Print and shaded views of the part. All mm, measured from the part's lowest x, y and z. A direction names the side the tool comes from. Give positions to 0.01 mm unless a question says otherwise; leave off trailing zeros. Loops run counter-clockwise (first coordinate to the right, second up) from the corner with the lowest first, then second, coordinate; pieces in that order, holes last. Notation, with made-up numbers: M 63.5,62.5 L 90.5,62.5 A22 cw 90.5,99.5 Z; hole C -31,5 d2. An arc over 180 degrees is marked long. Put each result on its own line as item: value. Start each with the question number.
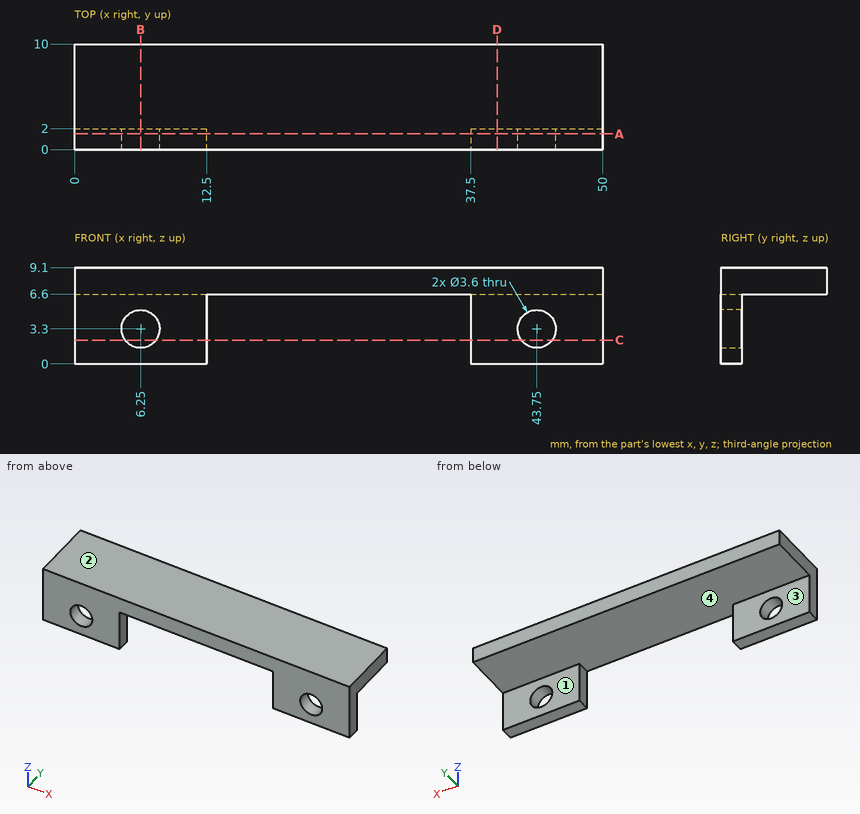
1) Band-saw the part on A-A on y = 1.5. Give the cut face in (x, z).
2) Band-saw the part on D-D on x = 40. Give the cut face in (y, z).
3) Band-saw the part on B-B on x = 6.25. Give the cut face in (y, z).
4) Band-saw the part on C-C on z = 2.25. Give the cut face in (x, y).
5) Wall check: L1, parallel to X at y = 1, z = 6; L2, parallel to Z at x = 6.5, y = 6.75; L3, parallel to Y at x = 4.5, z = 5.75. Give the ranges that are in metal, low to high.
6) Pin check, flat tips, straight feed: pin 1 Ø3 at (x, y) = (19.5, 5) entering from -Z; pin 2 Ø2 at (x, z) = (45, 2.5) entering from +Y. Stop position of each tip, or through.
7) Mould opens along X. For the marked faces 3 and 4 say: +X half, -X half, draft (parallel to the pull), parting line (faces both ways), or undercut.
8) Which spindle directions (+Z, -Z, +X, -X, +Y, -Y) get a long thin tool onto all of the face, cutting with end or side? Do the marked faces 1 and 2. Say none if no direction does.
Evaluation:
1. outline: M 0,0 L 12.5,0 L 12.5,6.6 L 37.5,6.6 L 37.5,0 L 50,0 L 50,9.1 L 0,9.1 Z; hole C 6.25,3.3 d3.6; hole C 43.75,3.3 d3.6
2. outline: M 0,0 L 2,0 L 2,6.6 L 10,6.6 L 10,9.1 L 0,9.1 Z
3. outline: M 0,0 L 2,0 L 2,1.5 L 0,1.5 Z; M 0,5.1 L 2,5.1 L 2,6.6 L 10,6.6 L 10,9.1 L 0,9.1 Z
4. outline: M 0,0 L 4.79,0 L 4.79,2 L 0,2 Z; M 7.71,0 L 12.5,0 L 12.5,2 L 7.71,2 Z; M 37.5,0 L 42.29,0 L 42.29,2 L 37.5,2 Z; M 45.21,0 L 50,0 L 50,2 L 45.21,2 Z
5. L1: 0 to 12.5, 37.5 to 50
5. L2: 6.6 to 9.1
5. L3: 0 to 2
6. pin 1: z = 6.6
6. pin 2: y = 2
7. face 3: draft
7. face 4: undercut
8. face 1: -Z, +X, -X, +Y
8. face 2: +Z, +X, -X, +Y, -Y
